Build history of the part. All positions in model axes, mm. Give positions to 0.01 mm unless a question says otherwise; leave off trailing zeros. Order: outer loops, then holes, each group sorted by start corner. A loop starts at its lowest first (then second) coordinate and runs counter-clockwise, first axis right, second up. Notation, with made-up numbers: (-29.75, 84.25) - (5.25, 84.25) arc R15 cw to (5.25, 103.25) - close; hole circle Ø11 at (-6, 32). An arc over 180 degrees is marked (long way). Use a Markdown table: item, result.
Autodesk Inventor part; units mm, degrees
ref_plane "YZ Plane" through (0, 0, 0) normal (1, 0, 0) x (0, 1, 0)
ref_plane "XZ Plane" through (0, 0, 0) normal (0, 1, 0) x (-1, 0, 0)
ref_plane "XY Plane" through (0, 0, 0) normal (0, 0, 1) x (1, 0, 0)
sketch "Sketch1" plane through (0, 0, 0) normal (0, 0, 1) x (1, 0, 0)
  circle A0 centre (-32.198, -0.1238) radius 50.8
  circle A1 centre (123.0816, -9.7192) radius 50.8
  arc A2 (-30.1614, 32.8334) -> (-34.2345, -33.0809) centre (-32.198, -0.1238) ccw
  arc A3 (121.045, -42.6763) -> (125.1181, 23.238) centre (123.0816, -9.7192) ccw
  line L0 (121.045, -42.6763) -> (-34.2345, -33.0809)
  line L1 (125.1181, 23.238) -> (-30.1614, 32.8334)
  arc A4 (120.8492, -45.8453) -> (125.314, 26.4069) centre (123.0816, -9.7192) ccw
  line L2 (120.8492, -45.8453) -> (-34.4304, -36.2499)
  arc A5 (-29.9656, 36.0023) -> (-34.4304, -36.2499) centre (-32.198, -0.1238) ccw
  line L3 (-29.9656, 36.0023) -> (125.314, 26.4069)
  point P0 (0, 0)
  dimension "d0" = 66.04
  dimension "d1" = 66.04
  dimension "d2" = 3.175
extrude "Extrusion1" add sketch "Sketch1" along normal mid plane 12.7 contours L1 A2 L0 A0 L2 A5 L3 | A0 L3 A1 L1 | L0 A1 L2 A0 | A1 L3 A4 L2 L0 A3 L1
properties part number "Belt"
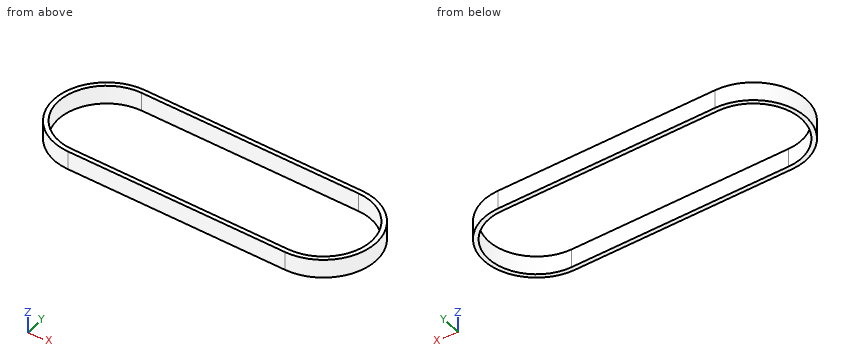
1) Slice it at C-C (x = -45.5). Write the cut outline in (y, z).
Computed:
| item | result |
|---|---|
| outline | (-33.79, -6.35) - (-30.35, -6.35) - (-30.35, 6.35) - (-33.79, 6.35) - close; (30.1, -6.35) - (33.54, -6.35) - (33.54, 6.35) - (30.1, 6.35) - close |
2) Slice it at B-B (y = 20.5). Write the cut outline in (x, z).
Computed:
| item | result |
|---|---|
| outline | (-61.94, -6.35) - (-57.99, -6.35) - (-57.99, 6.35) - (-61.94, 6.35) - close; (136.39, -6.35) - (143, -6.35) - (143, 6.35) - (136.39, 6.35) - close |
3) Pin check, flat tips, straight feed: P1, Ø1, axis at y = -36, z = 3, coming from the +X side; P2, Ø1.5, axis at y = 12.5, z = -4, coming from the -X side; P3, Ø3, axis at y = 8.5, z = 0.5, coming from the +X side. Stop position of each tip, or through.
Computed:
| item | result |
|---|---|
| P1 | stops at x = 148.49 |
| P2 | stops at x = -66.39 |
| P3 | stops at x = 155.18 |
4) Wall check: line 1 (X direction, y = -24, z = -3); line 2 (Y direction, x = -9.5, z = -1); line 3 (X direction, y = 19, z = 2.25). Give the ranges that are in metal, low to high. Write a range as from..to.
Computed:
| item | result |
|---|---|
| line 1 | x = -59.4..-55.01, 152.85..156.34 |
| line 2 | y = -37.79..-34.61, 31.56..34.74 |
| line 3 | x = -62.93..-59.12, 139.38..145.11 |
